Part print with two shaded views. Sizes in mm from the minimum x, y, z corner. A direction names the side the tool comes from. Round coordinates to 2 decimals unless told otherwise and drop trailing zeros. Write each loop counter-clockwise with the first axis right and the second up, starting at its lowest first coordinate (ties: lowest second). Pieces come first, ordered by that corner, then holes. Notation, with made-up numbers: (14, 41) -> (32, 41) arc R21 cw to (32, 64) -> close; hole circle Ø7 at (70.5, -17.75). An arc over 180 degrees is marked (long way). Return JSON: item names as keys, results as strings. Group by question number.
(1) Saw through at A-A (x = 30). List the corners of the cut face in (y, z), plus the area to 3 significant figures.
(2) Tool access for the marked faces 1, 2 and 3: list every direction of +Z, -Z, +X, -X, +Y, -Y with a clear straight run to the whole face (end or side of a thin tool).
(3) Mould opens along Y. For the marked faces 4, 5, 6 and 7 say: +Y half, -Y half, draft (parallel to the pull), parting line (faces both ways), or undercut.
(4) Saw through at D-D (z = 2). List the corners of the cut face in (x, y), plus the area to 3 significant figures.
(5) Saw through at B-B (z = 15). List the corners of the cut face in (x, y), plus the area to 3 significant figures.
(6) Saw through at C-C (y = 28). List the corners of the cut face in (x, z), plus the area to 3 significant figures.
(7) Drill centre lines: L1, parallel to Y at x = 10, z = 28; L2, parallel to Z at x = 14, y = 27; L3, parallel to X at y = 32, z = 23.25. Where is each one in solid material? Low to high. Write a range as from..to.
(8) Drop flat-ended pins along their axis: pin 1 Ø5 at (x, z) = (38, 17.5) entering from +Y; pin 2 Ø10 at (y, z) = (21.5, 6.5) entering from +X; pin 3 Ø6 at (x, z) = (20.5, 21.5) entering from +Y. Give the stop position or say it passes through.
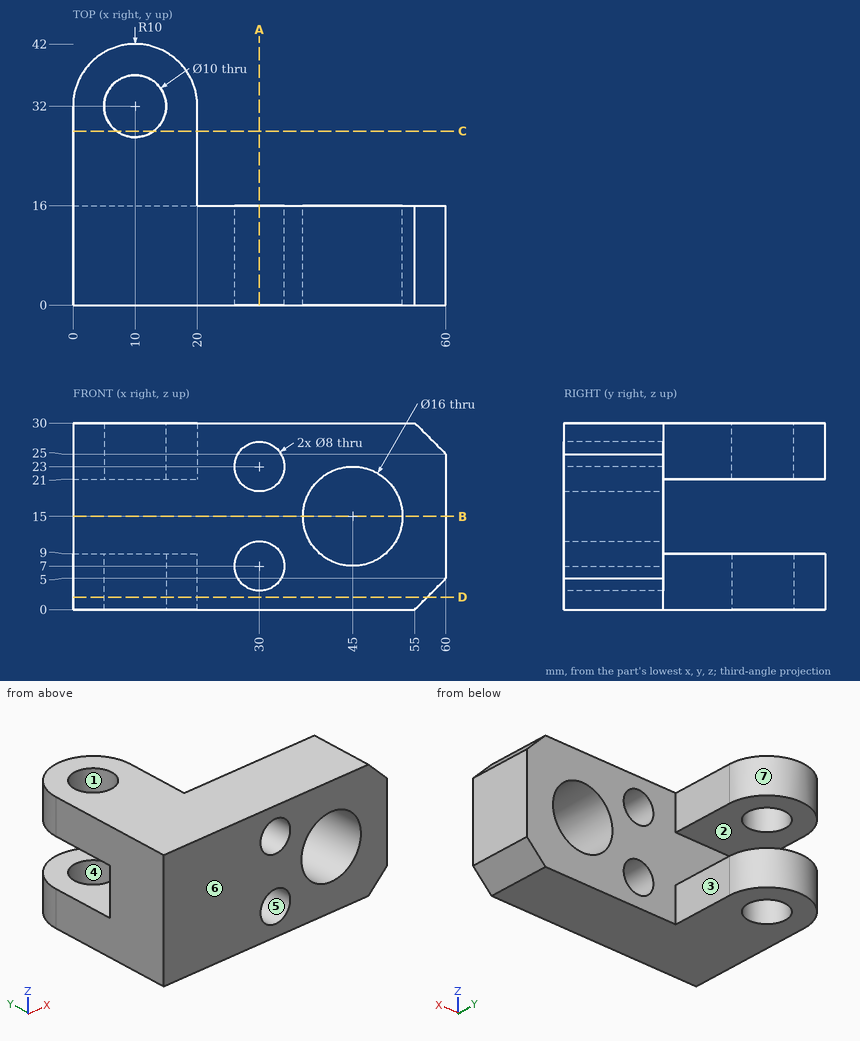
Computed values:
{
 "1": {"outline": "(0, 0) -> (16, 0) -> (16, 3) -> (0, 3) -> close; (0, 11) -> (16, 11) -> (16, 19) -> (0, 19) -> close; (0, 27) -> (16, 27) -> (16, 30) -> (0, 30) -> close", "area": "224 mm2"},
 "2": {"face 1": "+Z, -Z", "face 2": "+X, -X, +Y", "face 3": "+Z, -Z, +X, +Y"},
 "3": {"face 4": "undercut", "face 5": "draft", "face 6": "-Y half", "face 7": "+Y half"},
 "4": {"outline": "(0, 0) -> (57, 0) -> (57, 16) -> (20, 16) -> (20, 32) arc R10 ccw to (0, 32) -> close; hole circle Ø10 at (10, 32)", "area": "1,310 mm2"},
 "5": {"outline": "(0, 0) -> (37, 0) -> (37, 16) -> (0, 16) -> close; (53, 0) -> (60, 0) -> (60, 16) -> (53, 16) -> close", "area": "704 mm2"},
 "6": {"outline": "(0, 0) -> (7, 0) -> (7, 9) -> (0, 9) -> close; (0, 21) -> (7, 21) -> (7, 30) -> (0, 30) -> close; (13, 0) -> (20, 0) -> (20, 9) -> (13, 9) -> close; (13, 21) -> (20, 21) -> (20, 30) -> (13, 30) -> close", "area": "252 mm2"},
 "7": {"L1": "0..27, 37..42", "L2": "0..9, 21..30", "L3": "0..5, 15..20"},
 "8": {"pin 1": "y = 16", "pin 2": "x = 20", "pin 3": "y = 38.61"}
}
